from build123d import *

# Parameters (mm, degrees)
SKETCH1_W           = 25.4
SKETCH1_H           = 50.8
SKETCH1_W_2         = 22.225
SKETCH1_H_2         = 47.625
BOSS_EXTRUDE1_DEPTH = 50.8
SKETCH2_R           = 2.413
CUT_EXTRUDE1_DEPTH  = 77.2
SKETCH3_R           = 14.2875
CUT_EXTRUDE2_DEPTH  = 77.2


with BuildPart() as part:
    # Sketch1 → Boss-Extrude1 (new body)
    with BuildSketch(Plane.XY):
        with Locations((12.7, 25.4)):
            Rectangle(SKETCH1_W, SKETCH1_H)
        with Locations((12.7, 25.4)):
            Rectangle(SKETCH1_W_2, SKETCH1_H_2, mode=Mode.SUBTRACT)
    extrude(amount=BOSS_EXTRUDE1_DEPTH)

    # Sketch2 → Cut-Extrude1 (cut, through all)
    with BuildSketch(Plane(origin=(0, 50.8, 0), x_dir=(1, 0, 0), z_dir=(0, 1, 0))):
        with Locations(Location((12.7, -12.7, 0), (0, 0, 270))):
            Circle(SKETCH2_R)
        with Locations(Location((12.7, -38.1, 0), (0, 0, 270))):
            Circle(SKETCH2_R)
    extrude(amount=-CUT_EXTRUDE1_DEPTH, mode=Mode.SUBTRACT)

    # Sketch3 → Cut-Extrude2 (cut, through all)
    with BuildSketch(Plane(origin=(25.4, 0, 0), x_dir=(0, 0, -1), z_dir=(1, 0, 0))):
        with Locations((-25.4, 25.4)):
            Circle(SKETCH3_R)
    extrude(amount=-CUT_EXTRUDE2_DEPTH, mode=Mode.SUBTRACT)


solid = part.part
Here's how the part is built. I have some questions about the finished solid (model axes, mm). A direction names the side the tool comes from. Round coordinates to 2 decimals unless told otherwise and drop trailing zeros. Loops run counter-clockwise (first coordinate to the right, second up) from the corner with the lowest first, then second, coordinate; pieces in that order, holes last.
1. We'd pull the mould along Z, two halves only. Please class faces 1 (the face through (11.78, 0.8, 40.33)), 2 (the face through (13, 49.212, 25)), 3 (the face through (1, 27, 50.8)): +Z half, -Z half, draft (parallel to the pull), parting line (faces both ways), or undercut.
Answer list:
face 1: undercut
face 2: draft
face 3: +Z half
2. If we section it at C-C on x = 5.75: Write out the boundary of the cut face in (y, z), plus the area to 3 significant figures.
Answer list:
outline: (0, 0) - (1.59, 0) - (1.59, 50.8) - (0, 50.8) - close; (49.21, 0) - (50.8, 0) - (50.8, 50.8) - (49.21, 50.8) - close
area: 161 mm2
3. Which directions (+Z, -Z, +X, -X, +Y, -Y) give clear straight access to the entire face, cutting with the end or side of a thin tool? Please do faces 4 (the face through (10.344, 0.805, 12.177)), 5 (the face through (23.812, 36, 14)).
Answer list:
face 4: +Y, -Y
face 5: +Z, -Z
4. If we section it at B-B on z = 25.4: Write out the boundary of the cut face in (x, y), plus the area to 3 significant figures.
Answer list:
outline: (0, 0) - (25.4, 0) - (25.4, 11.11) - (23.81, 11.11) - (23.81, 1.59) - (1.59, 1.59) - (1.59, 11.11) - (0, 11.11) - close; (0, 39.69) - (1.59, 39.69) - (1.59, 49.21) - (23.81, 49.21) - (23.81, 39.69) - (25.4, 39.69) - (25.4, 50.8) - (0, 50.8) - close
area: 141 mm2
5. If we section it at A-A on y = 25.4: Write out the boundary of the cut face in (x, z), plus the area to 3 significant figures.
Answer list:
outline: (0, 0) - (1.59, 0) - (1.59, 11.11) - (0, 11.11) - close; (0, 39.69) - (1.59, 39.69) - (1.59, 50.8) - (0, 50.8) - close; (23.81, 0) - (25.4, 0) - (25.4, 11.11) - (23.81, 11.11) - close; (23.81, 39.69) - (25.4, 39.69) - (25.4, 50.8) - (23.81, 50.8) - close
area: 70.6 mm2
6. If we section it at D-D on y = 45.5: Write out the boundary of the cut face in (x, z), plus the area to 3 significant figures.
Answer list:
outline: (0, 0) - (1.59, 0) - (1.59, 50.8) - (0, 50.8) - close; (23.81, 0) - (25.4, 0) - (25.4, 50.8) - (23.81, 50.8) - close
area: 161 mm2
7. If I drill on line 1 along Y through (x, z) = (6.25, 25); line 2 along X through (y, z) = (49.9, 38.1); line 3 along X through (y, z) = (20, 46), over which ranges is the centre line in solid material (lowest first)?
Answer list:
line 1: y = 0 to 1.59, 49.21 to 50.8
line 2: x = 0 to 10.29, 15.11 to 25.4
line 3: x = 0 to 1.59, 23.81 to 25.4
